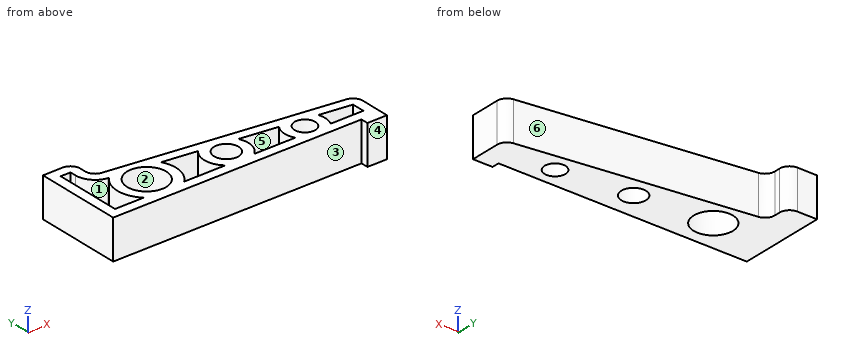
from build123d import *

# Parameters (mm, degrees)
F1_DEPTH    = 8
F2_R        = 2
F3_R        = 4
F3_R_2      = 2.5
F3_R_3      = 2.125
F4_DEPTH    = 8.001
F5_T        = 2
F5_T3_DEPTH = 12


# Not quite as in the source:
# - a shell that OpenCascade refuses in one call is made with other operations: the cavity is built on its own and cut out


with BuildPart() as f1:
    # F0 (on Top) → F1 (new body)
    with BuildSketch(Plane.XY):
        Polygon((-27.375, -6.35), (23.375, -6.35), (23.375, -7.85), (27.375, -7.85), (27.375, -6.35), (27.375, 0), (-21.375, 6.35), (-21.375, 11.35), (-27.375, 11.35), (-27.375, 6.35), align=None)
    extrude(amount=F1_DEPTH)

    # F2
    f2_edges = [f1.edges().sort_by_distance(p)[0] for p in [
        (-21.375, 11.35, 4),
        (27.375, 0, 4),
        (-21.375, 6.35, 4),
    ]]
    fillet(f2_edges, radius=F2_R)

    # F3 (on face) → F4 (cut, through all)
    with BuildSketch(Plane.XY.offset(8)):
        with Locations((-15.375, 0)):
            Circle(F3_R)
        with Locations((0.125, -0.9643055964)):
            Circle(F3_R_2)
        with Locations((15.0608578937, -2.35)):
            Circle(F3_R_3)
    extrude(amount=-F4_DEPTH, mode=Mode.SUBTRACT)

    # F5: shell of thickness 2, made by hand


with BuildPart() as f5_core1:
    # F5_t2: copy of F1
    add(f1.part)

    # the walls: a layer under each face that stays
    f5_faces = [f5_core1.faces().sort_by_distance(p)[0] for p in [
        (27.375, -4.8031912743, 4),
        (25.375, -7.85, 4),
        (3, 3.175, 4),
        (23.375, -7.1, 4),
        (-20.8777742764, 6.7866592918, 4),
        (-2, -6.35, 4),
        (-21.375, 8.7281912743, 4),
        (-27.375, 2.5, 4),
        (-25.375, 11.35, 4),
        (-2.375, -0.9643055964, 4),
        (12.9358578937, -2.35, 4),
        (-19.375, 0, 4),
        (0, 1.75, 0),
    ]]
    thicken(f5_faces, amount=-F5_T, mode=Mode.SUBTRACT)

    # F5_s4 → F5_t3 (cut)
    with BuildSketch(Plane.XY.offset(-2)):
        Polygon((23.355, -6.37), (25.375, -6.35), (25.375, -4.35), (23.375, -4.35), align=None)
    extrude(amount=F5_T3_DEPTH, mode=Mode.SUBTRACT)


with BuildPart() as f1_1:
    add(f1.part)

    # what is left inside the walls is the cavity
    f5_cavity = [f5_core1.part.solids().sort_by_distance(p)[0] for p in [
        (22.021788, -4.33, 6),
        (7.27122, -4.33, 6),
        (-25.355, 2.5, 6),
        (-7.040903, -4.33, 6),
    ]]
    add(f5_cavity, mode=Mode.SUBTRACT)


solid = f1_1.part
The listing builds one solid part. Answer for the finished solid, in the listing's coordinates (mm). Face numbers are marked on the shaded views. A direction names the side the tool comes from. Round coordinates to 2 decimals unless told otherwise and drop trailing zeros. Order: outer loops, then holes, each group sorted by start corner. A loop starts at its lowest first (then second) coordinate and runs counter-clockwise, first axis right, second up. Notation, with made-up numbers: (-30, 45.25) -> (-16, 45.25) arc R19 ccw to (-16, 52.25) -> close; hole circle Ø2 at (19.25, 55.5). An arc over 180 degrees is marked (long way). One line per item, written item: value.
Item 1: Find section B-B, the plane y = -2.35. State how many separate pieces and enclosed holes the cut face has, then the cut area to 3 significant figures.
Taken from the geometry:
separate pieces: 4
enclosed holes: 0
area: 182 mm2
Item 2: For the marked faces 1, 2 and 3, determine the directions among +Z, -Z, +X, -X, +Y, -Y from which every point of the face is accessible in a straight line to the end or side of a thin tool.
Taken from the geometry:
face 1: +Z
face 2: +Z, -Z
face 3: +Z, -Z, -X, -Y
Item 3: Given P1, Ø1.5, axis at x = 4.5, z = 3, coming from the -Y side; P2, Ø1.8, axis at y = 0.5, z = 4, coming from the +X side; P3, Ø3, axis at x = -6, z = 4, coming from the +Y side; P4, Ø2.5, axis at x = 15.06, y = -2.35, coming from the +Z side, each flat-ended and moving along its own axis, determine where each tip first touches the part or whether it passes through.
Taken from the geometry:
P1: stops at y = -6.35
P2: stops at x = 26.84
P3: stops at y = 4.54
P4: passes through
Item 4: For a pull along X with two mould halves and no side action, classify the marked faces 4, 5 and 6 as released by +X, released by -X, zero draft, split by the parting line, or undercut.
Taken from the geometry:
face 4: zero draft
face 5: undercut
face 6: released by +X
Item 5: Straight lines are drawn through the part: L1, parallel to X at y = 9, z = 7 (3 decimals); L2, parallel to Y at x = 6.5, z = 2.75; L3, parallel to Y at x = 7.5, z = 7.5. For each, find the intervals that lie inside material, in ascending order.
Taken from the geometry:
L1: x = -27.375 to -25.375, -23.375 to -21.375
L2: y = -6.35 to -4.35, 0.7 to 2.72
L3: y = -6.35 to -4.35, 0.57 to 2.59
Item 6: Find section A-A, the plane x = -24. Give the vertices of the cut face in (y, z), then the cut area to 3 significant figures.
Taken from the geometry:
outline: (-6.35, 0) -> (11.35, 0) -> (11.35, 8) -> (9.35, 8) -> (9.35, 2) -> (-4.35, 2) -> (-4.35, 8) -> (-6.35, 8) -> close
area: 59.4 mm2
